Read the model definition and answer for the solid it produces. Units are mm, in the model's axes. A direction names the side the tool comes from. Give positions to 0.01 mm unless a question says otherwise; leave off trailing zeros. Write each loop counter-clockwise with the first axis right and the second up, starting at its lowest first coordinate (ties: lowest second). Pieces come first, ordered by that corner, then holes. Notation, with made-up numbers: (71.5, 58.5) -> (97.5, 58.5) arc R26 cw to (97.5, 89.5) -> close; hole circle Ø1 at (80, -34). An arc over 180 degrees is marked (long way). Write item = value, one per line.
from build123d import *

# Parameters (mm, degrees)
SKETCH1_R                = 68.369999998
SKETCH1_R_2              = 23.401
BOSS_EXTRUDE1_DEPTH      = 2
BOSS_EXTRUDE2_START      = -13
SKETCH3_R                = 68.369999998
SKETCH3_R_2              = 66.37
BOSS_EXTRUDE2_DEPTH      = 13
CUT_EXTRUDE40_DEPTH      = 114.575806629
CUT_EXTRUDE40_DEPTH_BACK = 114.575806629
SKETCH63_R               = 2
CUT_EXTRUDE41_DEPTH      = 160.130961581
CUT_EXTRUDE41_DEPTH_BACK = 160.130961581
SKETCH64_R               = 2
CUT_EXTRUDE45_DEPTH      = 2
SKETCH73_R               = 1
CUT_EXTRUDE47_DEPTH      = 10
SKETCH70_R               = 1.5
CUT_EXTRUDE48_DEPTH      = 10
SKETCH74_R               = 5
CUT_EXTRUDE49_DEPTH      = 10
CUT_EXTRUDE51_START      = -2
CUT_EXTRUDE51_DEPTH      = 2
SKETCH80_R               = 5
SKETCH80_R_2             = 1.5
SKETCH80_R_3             = 1
SKETCH80_R_4             = 23.401
BOSS_EXTRUDE4_DEPTH      = 2


with BuildPart() as part:
    # Sketch1 → Boss-Extrude1 (new body)
    with BuildSketch(Plane(origin=(0, 0, 0), x_dir=(-0.9985653746512714, 0, -0.053546172109368295), z_dir=(0, 1, 0))):
        with Locations(Location((55.498672647, -32.344920806, 0), (0, 0, 93.069437642))):
            Circle(SKETCH1_R)
        with Locations(Location((55.498672647, -32.344920806, 0), (0, 0, 93.069437642))):
            Circle(SKETCH1_R_2, mode=Mode.SUBTRACT)
    extrude(amount=BOSS_EXTRUDE1_DEPTH)

    # Sketch3 → Boss-Extrude2 (add)
    with BuildSketch(Plane(origin=(0, 2, 0), x_dir=(1, 0, 0), z_dir=(0, 1, 0)).offset(BOSS_EXTRUDE2_START)):
        with Locations(Location((-53.687106148, 35.27025944, 0), (0, 0, 270))):
            Circle(SKETCH3_R)
        with Locations(Location((-53.687106148, 35.27025944, 0), (0, 0, 270))):
            Circle(SKETCH3_R_2, mode=Mode.SUBTRACT)
    extrude(amount=BOSS_EXTRUDE2_DEPTH)

    # Sketch63 → Cut-Extrude40 (cut, two sides: drawn at the far end of the back side and taken through both)
    with BuildSketch(Plane(origin=(-41.506941316, 0, -46.21062949), x_dir=(0.7439552092791144, 2.284460434874975e-13, -0.6682294864688846), z_dir=(0.6682294864688846, -2.5433421830845933e-13, 0.7439552092791144)).offset(-CUT_EXTRUDE40_DEPTH_BACK)):
        with Locations((-16.372174937, -4.35)):
            Circle(SKETCH63_R)
    extrude(amount=CUT_EXTRUDE40_DEPTH + CUT_EXTRUDE40_DEPTH_BACK, mode=Mode.SUBTRACT)

    # Sketch64 → Cut-Extrude41 (cut, two sides: drawn at the far end of the back side and taken through both)
    with BuildSketch(Plane(origin=(-12.180164832, 0, 10.94037005), x_dir=(-0.668229486468876, 1.5883353274739987e-15, -0.743955209279122), z_dir=(0.743955209279122, -1.7683301393964735e-15, -0.668229486468876)).offset(-CUT_EXTRUDE41_DEPTH_BACK)):
        with Locations((62.114800614, -4.35)):
            Circle(SKETCH64_R)
    extrude(amount=CUT_EXTRUDE41_DEPTH + CUT_EXTRUDE41_DEPTH_BACK, mode=Mode.SUBTRACT)

    # Sketch67 → Cut-Extrude45 (cut)
    with BuildSketch(Plane(origin=(0, 2, 0), x_dir=(1, 0, 0), z_dir=(0, 1, 0))):
        with BuildLine():
            Line((-47.831144931, 125.709400378), (-49.82827568, 125.816492726))
            Line((-49.82827568, 125.816492726), (-52.215508738, 81.297751413))
            ThreePointArc((-52.215508738, 81.297751413), (-51.270489538, 80.245639864), (-50.218377989, 81.190659065))
            Line((-50.218377989, 81.190659065), (-47.831144931, 125.709400378))
        make_face()
        with BuildLine():
            Line((-144.126247086, 41.126220657), (-144.233339434, 39.129089908))
            Line((-144.233339434, 39.129089908), (-99.714598121, 36.741856849))
            ThreePointArc((-99.714598121, 36.741856849), (-98.662486572, 37.68687605), (-99.607505773, 38.738987598))
            Line((-99.607505773, 38.738987598), (-144.126247086, 41.126220657))
        make_face()
        with BuildLine():
            Line((36.75203479, 29.414298222), (36.859127139, 31.411428971))
            Line((36.859127139, 31.411428971), (-7.659614175, 33.79866203))
            ThreePointArc((-7.659614175, 33.79866203), (-8.711725723, 32.853642829), (-7.766706523, 31.801531281))
            Line((-7.766706523, 31.801531281), (36.75203479, 29.414298222))
        make_face()
    extrude(amount=-CUT_EXTRUDE45_DEPTH, mode=Mode.SUBTRACT)

    # Sketch73 → Cut-Extrude47 (cut)
    with BuildSketch(Plane.XZ.offset(-2)):
        with Locations(Location((-72.2141021, -18.632644766, 0), (0, 0, 90))):
            Circle(SKETCH73_R)
        with Locations(Location((-37.049491474, -16.743263487, 0), (0, 0, 90))):
            Circle(SKETCH73_R)
        with Locations(Location((-35.160110195, -51.907874114, 0), (0, 0, 90))):
            Circle(SKETCH73_R)
        with Locations(Location((-70.324720822, -53.797255392, 0), (0, 0, 90))):
            Circle(SKETCH73_R)
    extrude(amount=CUT_EXTRUDE47_DEPTH, mode=Mode.SUBTRACT)

    # Sketch70 → Cut-Extrude48 (cut)
    with BuildSketch(Plane(origin=(0, 2, 0), x_dir=(1, 0, 0), z_dir=(0, 1, 0))):
        with Locations(Location((-99.774462502, 65.286181619, 0), (0, 0, 270))):
            Circle(SKETCH70_R)
        with Locations(Location((-56.637979096, -19.650523046, 0), (0, 0, 270))):
            Circle(SKETCH70_R)
        with Locations(Location((-4.648876845, 60.175119746, 0), (0, 0, 270))):
            Circle(SKETCH70_R)
    extrude(amount=-CUT_EXTRUDE48_DEPTH, mode=Mode.SUBTRACT)

    # Sketch74 → Cut-Extrude49 (cut)
    with BuildSketch(Plane(origin=(19.562495047, 3, -2.053609117), x_dir=(1, 0, 0), z_dir=(0, 1, 0))):
        with Locations(Location((-105.702188225, 2.042468777, 0), (0, 0, 270))):
            Circle(SKETCH74_R)
        with Locations(Location((-44.324158759, -1.255349618, 0), (0, 0, 270))):
            Circle(SKETCH74_R)
    extrude(amount=-CUT_EXTRUDE49_DEPTH, mode=Mode.SUBTRACT)

    # Sketch75 → Cut-Extrude51 (cut)
    with BuildSketch(Plane(origin=(0, 2, 0), x_dir=(1, 0, 0), z_dir=(0, 1, 0)).offset(CUT_EXTRUDE51_START)):
        with BuildLine():
            ThreePointArc((-78.28711428, 99.061297209), (-79.21750955, 98.694666428), (-80.142442845, 98.314466628))
            Line((-80.142442845, 98.314466628), (-79.765783898, 97.378744227))
            Line((-79.765783898, 97.378744227), (-71.802851111, 77.596671772))
            ThreePointArc((-71.802851111, 77.596671772), (-70.501771538, 77.04242278), (-69.947522546, 78.343502353))
            Line((-69.947522546, 78.343502353), (-77.910455333, 98.125574808))
            Line((-77.910455333, 98.125574808), (-78.28711428, 99.061297209))
        make_face()
        with BuildLine():
            Line((-21.107609811, 94.229039398), (-20.63291657, 95.119047657))
            ThreePointArc((-20.63291657, 95.119047657), (-21.511818593, 95.596106061), (-22.397604199, 96.060258351))
            Line((-22.397604199, 96.060258351), (-22.872297441, 95.170250092))
            Line((-22.872297441, 95.170250092), (-32.907769586, 76.354618611))
            ThreePointArc((-32.907769586, 76.354618611), (-32.496031118, 75.00166945), (-31.143081956, 75.413407918))
            Line((-31.143081956, 75.413407918), (-21.107609811, 94.229039398))
        make_face()
        with BuildLine():
            Line((-76.23113034, -4.872889039), (-86.266602485, -23.688520519))
            Line((-86.266602485, -23.688520519), (-86.741295726, -24.578528778))
            ThreePointArc((-86.741295726, -24.578528778), (-85.862393702, -25.055587182), (-84.976608096, -25.519739471))
            Line((-84.976608096, -25.519739471), (-84.501914855, -24.629731212))
            Line((-84.501914855, -24.629731212), (-74.46644271, -5.814099732))
            ThreePointArc((-74.46644271, -5.814099732), (-74.878181178, -4.461150571), (-76.23113034, -4.872889039))
        make_face()
        with BuildLine():
            Line((-29.463756963, -27.585055929), (-29.087098016, -28.52077833))
            ThreePointArc((-29.087098016, -28.52077833), (-28.156702745, -28.154147549), (-27.231769451, -27.773947749))
            Line((-27.231769451, -27.773947749), (-27.608428398, -26.838225348))
            Line((-27.608428398, -26.838225348), (-35.571361185, -7.056152893))
            ThreePointArc((-35.571361185, -7.056152893), (-36.872440758, -6.501903901), (-37.42668975, -7.802983474))
            Line((-37.42668975, -7.802983474), (-29.463756963, -27.585055929))
        make_face()
    extrude(amount=CUT_EXTRUDE51_DEPTH, mode=Mode.SUBTRACT)

    # Sketch80 → Boss-Extrude4 (add)
    with BuildSketch(Plane(origin=(0, 2, 0), x_dir=(1, 0, 0), z_dir=(0, 1, 0))):
        with BuildLine():
            Line((-29.087098016, -28.52077833), (-37.42668975, -7.802983474))
            ThreePointArc((-37.42668975, -7.802983474), (-36.872440758, -6.501903901), (-35.571361185, -7.056152893))
            Line((-35.571361185, -7.056152893), (-27.231769451, -27.773947749))
            ThreePointArc((-27.231769451, -27.773947749), (1.922948187, -4.503837114), (14.523625835, 30.606254489))
            Line((14.523625835, 30.606254489), (-7.766706523, 31.801531281))
            ThreePointArc((-7.766706523, 31.801531281), (-8.711725723, 32.853642829), (-7.659614175, 33.79866203))
            Line((-7.659614175, 33.79866203), (14.630861042, 32.603377578))
            ThreePointArc((14.630861042, 32.603377578), (5.862291778, 68.860825176), (-20.63291657, 95.119047657))
            Line((-20.63291657, 95.119047657), (-31.143081956, 75.413407918))
            ThreePointArc((-31.143081956, 75.413407918), (-32.496031118, 75.00166945), (-32.907769586, 76.354618611))
            Line((-32.907769586, 76.354618611), (-22.397604199, 96.060258351))
            ThreePointArc((-22.397604199, 96.060258351), (-35.331439872, 101.130159344), (-49.023101197, 103.480991422))
            Line((-49.023101197, 103.480991422), (-50.218377989, 81.190659065))
            ThreePointArc((-50.218377989, 81.190659065), (-51.270489538, 80.245639864), (-52.215508738, 81.297751413))
            Line((-52.215508738, 81.297751413), (-51.020224286, 103.588226629))
            ThreePointArc((-51.020224286, 103.588226629), (-64.884819285, 102.71703935), (-78.28711428, 99.061297209))
            Line((-78.28711428, 99.061297209), (-69.947522546, 78.343502353))
            ThreePointArc((-69.947522546, 78.343502353), (-70.501771538, 77.04242278), (-71.802851111, 77.596671772))
            Line((-71.802851111, 77.596671772), (-80.142442845, 98.314466628))
            ThreePointArc((-80.142442845, 98.314466628), (-109.297160483, 75.044355993), (-121.89783813, 39.93426439))
            Line((-121.89783813, 39.93426439), (-99.607505773, 38.738987598))
            ThreePointArc((-99.607505773, 38.738987598), (-98.662486572, 37.68687605), (-99.714598121, 36.741856849))
            Line((-99.714598121, 36.741856849), (-122.005073337, 37.937141302))
            ThreePointArc((-122.005073337, 37.937141302), (-113.236504074, 1.679693704), (-86.741295726, -24.578528778))
            Line((-86.741295726, -24.578528778), (-76.23113034, -4.872889039))
            ThreePointArc((-76.23113034, -4.872889039), (-74.878181178, -4.461150571), (-74.46644271, -5.814099732))
            Line((-74.46644271, -5.814099732), (-84.976608096, -25.519739471))
            ThreePointArc((-84.976608096, -25.519739471), (-57.353015371, -33.00138921), (-29.087098016, -28.52077833))
        make_face()
        with Locations(Location((-86.139693179, 4.096077895, 0), (0, 0, 270))):
            Circle(SKETCH80_R, mode=Mode.SUBTRACT)
        with Locations(Location((-99.774462502, 65.286181619, 0), (0, 0, 270))):
            Circle(SKETCH80_R_2, mode=Mode.SUBTRACT)
        with Locations(Location((-35.160110195, 51.907874114, 0), (0, 0, 270))):
            Circle(SKETCH80_R_3, mode=Mode.SUBTRACT)
        with Locations(Location((-53.687106148, 35.27025944, 0), (0, 0, 270))):
            Circle(SKETCH80_R_4, mode=Mode.SUBTRACT)
        with Locations(Location((-70.324720822, 53.797255392, 0), (0, 0, 270))):
            Circle(SKETCH80_R_3, mode=Mode.SUBTRACT)
        with Locations(Location((-37.049491474, 16.743263487, 0), (0, 0, 270))):
            Circle(SKETCH80_R_3, mode=Mode.SUBTRACT)
        with Locations(Location((-72.2141021, 18.632644766, 0), (0, 0, 270))):
            Circle(SKETCH80_R_3, mode=Mode.SUBTRACT)
        with Locations(Location((-56.637979096, -19.650523046, 0), (0, 0, 270))):
            Circle(SKETCH80_R_2, mode=Mode.SUBTRACT)
        with Locations(Location((-4.648876845, 60.175119746, 0), (0, 0, 270))):
            Circle(SKETCH80_R_2, mode=Mode.SUBTRACT)
        with Locations(Location((-24.761663712, 0.798259499, 0), (0, 0, 270))):
            Circle(SKETCH80_R, mode=Mode.SUBTRACT)
    extrude(amount=BOSS_EXTRUDE4_DEPTH)


solid = part.part
(1) Given P1, Ø8, axis at y = -3.5, z = -41.5, coming from the +X side; P2, Ø1.1, axis at x = -50, z = -102, coming from the +Y side; P3, Ø2.5, axis at x = -99.77, z = -65.29, coming from the +Y side; P4, Ø8, axis at y = -3, z = -76.5, coming from the -X side, each flat-ended and moving along its own axis, determine where each tip first touches the part or whether it passes through.
Checks:
P1 = 14.65
P2 = 0
P3 = through
P4 = -111.03
(2) The part is cut by section D-D on y = -8. Determine the outline of the cut face in (x, z).
Checks:
outline = circle Ø136.74 at (-53.69, -35.27); hole circle Ø132.74 at (-53.69, -35.27)
(3) The part is cut by section A-A on z = -2.5. Determine the outline of the cut face in (x, y).
Checks:
outline = (-113.69, -11) -> (-111.4, -11) -> (-111.4, 0) -> (-90.88, 0) -> (-90.88, 4) -> (-113.69, 4) -> close; (-81.4, 0) -> (-29.46, 0) -> (-29.46, 4) -> (-81.4, 4) -> close; (-20.06, 0) -> (4.03, 0) -> (4.03, -11) -> (6.32, -11) -> (6.32, 4) -> (-20.06, 4) -> close
(4) A tool of negligible diameter and unlimited length cuts with its end or side. For faces 1 (the flat face through (-53, 0, -7)), 2 (the cylindrical face through (-100.192, -4.262, -84.055)), from which of +Z, -Z, +X, -X, +Y, -Y can it reach the whole face along a straight path? Write none if from no direction.
Checks:
face_1 = -Y
face_2 = none
(5) For a pull along X with two mould halves and no side action, classify faces 3 (the flat face through (-24, 4, -36)), 4 (the flat face through (3.534, 1.972, -31.196)), 5 (the cylindrical face through (-94.07, -5.58, -87.94)) as released by +X, released by -X, zero draft, split by the parting line, or undercut.
Checks:
face_3 = zero draft
face_4 = released by +X
face_5 = undercut
(6) The part is cut by section B-B on x = -64. Determine the outline of the cut face in (y, z).
Checks:
outline = (-11, -102.86) -> (4, -102.86) -> (4, -56.28) -> (0, -56.28) -> (0, -100.83) -> (-11, -100.83) -> close; (-11, 30.29) -> (0, 30.29) -> (0, -14.26) -> (4, -14.26) -> (4, 32.32) -> (-11, 32.32) -> close
(7) Consider L1, parallel to X at y = 2.5, z = -1.5; L2, parallel to Z at x = -82, y = 2; L3, parallel to Y at x = -105, z = -39.5. Determine where each line is inside the solid, lowest interval first.
Checks:
L1 = -113.13 to -90.41, -81.87 to -29.71, -19.81 to 5.76
L2 = -97.5 to -6.9, -1.29 to 15.69, 19.94 to 26.96
L3 = 0 to 4
(8) The part is cut by section C-C on x = -15. Determine the outline of the cut face in (y, z), plus the area to 3 significant figures.
Checks:
outline = (-11, -91.64) -> (4, -91.64) -> (4, 21.1) -> (-11, 21.1) -> (-11, 18.66) -> (0, 18.66) -> (0, -89.2) -> (-11, -89.2) -> close
area = 505 mm²
